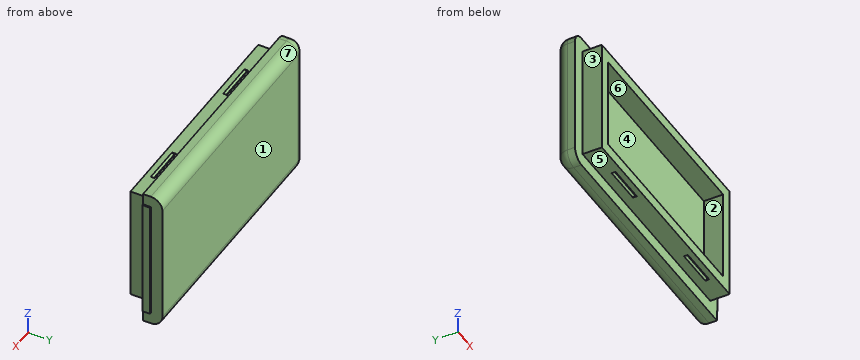
from build123d import *

# Parameters (mm, degrees)
SKETCH1_W           = 67
SKETCH1_H           = 37
BOSS_EXTRUDE2_DEPTH = 5
SKETCH1_4_W         = 60
SKETCH1_4_H         = 30
BOSS_EXTRUDE3_DEPTH = 10
CUT_EXTRUDE1_START  = -10
SKETCH1_6_W         = 54
SKETCH1_6_H         = 24
CUT_EXTRUDE1_DEPTH  = 5
FILLET1_R           = 3
CAVITY1_START       = -3
CAVITY1_OUTLINE_W   = 0.336287878
CAVITY1_OUTLINE_H   = 40
CAVITY1_DEPTH       = 3
CAVITY1_START_2     = -5
CAVITY1_2_DEPTH     = 2
CAVITY1_START_3     = -16.617009358
CAVITY1_3_OUTLINE_W = 10
CAVITY1_3_OUTLINE_H = 2.403805922
CAVITY1_3_DEPTH     = 0.707106781
CAVITY1_START_4     = 4.596194078
CAVITY1_4_OUTLINE_W = 10
CAVITY1_4_OUTLINE_H = 2.090097423
CAVITY1_4_DEPTH     = 0.707106781


# Read off the part's stored shape, not the designer's step: Cavity1
with BuildPart() as part:
    # Sketch1 → Boss-Extrude2 (new body)
    with BuildSketch(Plane(origin=(0, 0, 0), x_dir=(1, 0, 0), z_dir=(0, 1, 0))):
        Rectangle(SKETCH1_W, SKETCH1_H)
    extrude(amount=-BOSS_EXTRUDE2_DEPTH)

    # Sketch1<4> → Boss-Extrude3 (add)
    with BuildSketch(Plane(origin=(0, 0, 0), x_dir=(1, 0, 0), z_dir=(0, 1, 0))):
        Rectangle(SKETCH1_4_W, SKETCH1_4_H)
    extrude(amount=-BOSS_EXTRUDE3_DEPTH)

    # Sketch1<6> → Cut-Extrude1 (cut)
    with BuildSketch(Plane(origin=(0, 0, 0), x_dir=(1, 0, 0), z_dir=(0, 1, 0)).offset(CUT_EXTRUDE1_START)):
        Rectangle(SKETCH1_6_W, SKETCH1_6_H)
    extrude(amount=CUT_EXTRUDE1_DEPTH, mode=Mode.SUBTRACT)

    # Fillet1
    fillet1_edges = [part.edges().sort_by_distance(p)[0] for p in [
        (0, 0, -18.5),
        (0, 0, 18.5),
        (-33.5, 0, 0),
        (-33.5, -2.5, -18.5),
        (-33.5, -2.5, 18.5),
    ]]
    fillet(fillet1_edges, radius=FILLET1_R)

    # Cavity1 outline → Cavity1 (cut)
    with BuildSketch(Plane(origin=(0, 0, 0), x_dir=(1, 0, 0), z_dir=(0, 1, 0)).offset(CAVITY1_START)):
        with Locations((33.331856061, 0)):
            Rectangle(CAVITY1_OUTLINE_W, CAVITY1_OUTLINE_H)
    extrude(amount=CAVITY1_DEPTH, mode=Mode.SUBTRACT)

    # Cavity1 2 outline → Cavity1 2 (cut)
    with BuildSketch(Plane(origin=(0, 0, 0), x_dir=(1, 0, 0), z_dir=(0, 1, 0)).offset(CAVITY1_START_2)):
        with BuildLine():
            Line((33.163712122, -15.5), (33.163712122, -20))
            Line((33.163712122, -20), (33.5, -20))
            Line((33.5, -20), (33.5, -15.509431541))
            ThreePointArc((33.5, -15.509431541), (33.331922177, -15.502358349), (33.163712122, -15.5))
        make_face()
        with BuildLine():
            Line((33.163712122, 20), (33.163712122, 15.5))
            ThreePointArc((33.163712122, 15.5), (33.331922177, 15.502358349), (33.5, 15.509431541))
            Line((33.5, 15.509431541), (33.5, 20))
            Line((33.5, 20), (33.163712122, 20))
        make_face()
    extrude(amount=CAVITY1_2_DEPTH, mode=Mode.SUBTRACT)

    # Cavity1 3 outline → Cavity1 3 (cut)
    with BuildSketch(Plane(origin=(0, 0, 0), x_dir=(1, 0, 0), z_dir=(0, 0.70710678118654, 0.707106781186555)).offset(CAVITY1_START_3)):
        with Locations((18.163712122, 5.798097039)):
            Rectangle(CAVITY1_3_OUTLINE_W, CAVITY1_3_OUTLINE_H)
        with Locations((-15.836287878, 5.798097039)):
            Rectangle(CAVITY1_3_OUTLINE_W, CAVITY1_3_OUTLINE_H)
    extrude(amount=CAVITY1_3_DEPTH, mode=Mode.SUBTRACT)

    # Cavity1 4 outline → Cavity1 4 (cut)
    with BuildSketch(Plane(origin=(0, 0, 0), x_dir=(1, 0, 0), z_dir=(0, 0.70710678118654, 0.707106781186555)).offset(CAVITY1_START_4)):
        with Locations((18.163712122, -16.954951288)):
            Rectangle(CAVITY1_4_OUTLINE_W, CAVITY1_4_OUTLINE_H)
        with Locations((-15.836287878, -16.954951288)):
            Rectangle(CAVITY1_4_OUTLINE_W, CAVITY1_4_OUTLINE_H)
    extrude(amount=CAVITY1_4_DEPTH, mode=Mode.SUBTRACT)


solid = part.part
Geometry check sheet. Reference: the model listing, model coordinates, mm. Face numbers are marked on the shaded views. A direction names the side the tool comes from. Coordinates: 2 decimals unless noted, no trailing zeros. Order: outer loops, then holes, each group sorted by start corner. A loop starts at its lowest first (then second) coordinate and runs counter-clockwise, first axis right, second up. Notation, with made-up numbers: (80.25, 35.25) -> (96.25, 35.25) arc R22 cw to (96.25, 68.25) -> close; hole circle Ø10 at (35, 12). An arc over 180 degrees is marked (long way). Use a Markdown table: item, result. Add a question column.
1. Cross-section at D-D (x = -16). Enter the section's corners in (y, z).
2. Mould release check, pull along Z, two halves, no side actions. Record for the marked faces 4, 5, 6 and 7: pulls with the +Z half, pulls with the -Z half, needs draft (parallel to the pull), parting line crosses it, or undercut.
3. Cross-section at B-B (z = 13.5). Enter the section's corners in (x, y), and give its area (3 significant figures).
4. Cross-section at C-C (x = 1). Enter the section's corners in (y, z), and give its area (3 significant figures).
5. Material ranges on L1, parallel to X at y = -6.5, z = -8; L2, parallel to Z at x = -16, y = -6; L3, parallel to Y at x = 31, z = -10, recorded low to high.
6. Go/stop test with flat-tipped pins: pin 1 Ø5.5 at (y, z) = (-6.5, -6) entering from -X; pin 2 Ø0.5 at (y, z) = (-8, 14.5) entering from -X; pin 3 Ø4 at (x, z) = (12, -6) entering from -Y; pin 4 Ø2.5 at (x, y) = (5.5, -7.5) entering from -Z. Record where each tip stops, or that it passes through.
7. Cross-section at A-A (y = -5.75). Enter the section's corners in (x, z).
8. Set-up check for the marked faces 1, 2 and 3: record each of +Z, -Z, +X, -X, +Y, -Y from which the full face is reachable in a straight line by a thin tool's end or side.
Filled sheet:
| question | item | result |
|---|---|---|
| 1 | outline | (-10, -15) -> (-8.5, -15) -> (-8, -14.5) -> (-7.5, -15) -> (-5, -15) -> (-5, -18.5) -> (-3, -18.5) arc R3 ccw to (0, -15.5) -> (0, 15.5) arc R3 ccw to (-3, 18.5) -> (-5, 18.5) -> (-5, 15) -> (-7.5, 15) -> (-8, 14.5) -> (-8.5, 15) -> (-10, 15) -> (-10, 12) -> (-5, 12) -> (-5, -12) -> (-10, -12) -> close |
| 2 | face 4 | undercut |
| 2 | face 5 | pulls with the -Z half |
| 2 | face 6 | undercut |
| 2 | face 7 | pulls with the +Z half |
| 3 | outline | (-33.5, -5) -> (-30, -5) -> (-30, -10) -> (30, -10) -> (30, -5) -> (33.5, -5) -> (33.5, -3) -> (33.16, -3) -> (33.16, 0) -> (-30.5, 0) arc R3 ccw to (-33.5, -3) -> close |
| 3 | area | 632 mm2 |
| 4 | outline | (-10, -15) -> (-5, -15) -> (-5, -18.5) -> (-3, -18.5) arc R3 ccw to (0, -15.5) -> (0, 15.5) arc R3 ccw to (-3, 18.5) -> (-5, 18.5) -> (-5, 15) -> (-10, 15) -> (-10, 12) -> (-5, 12) -> (-5, -12) -> (-10, -12) -> close |
| 4 | area | 211 mm2 |
| 5 | L1 | -30 to -27, 27 to 30 |
| 5 | L2 | -15 to -12, 12 to 15 |
| 5 | L3 | -5 to 0 |
| 6 | pin 1 | x = -33.5 |
| 6 | pin 2 | x = -30 |
| 6 | pin 3 | y = -5 |
| 6 | pin 4 | z = -15 |
| 7 | outline | (-30, -15) -> (30, -15) -> (30, 15) -> (-30, 15) -> close; hole (-27, -12) -> (27, -12) -> (27, 12) -> (-27, 12) -> close |
| 8 | face 1 | +Z, -Z, +X, -X, +Y |
| 8 | face 2 | -Y |
| 8 | face 3 | +Z, -Z, -X, -Y |
